Model file for the job. Use its own axes, mm. Give positions to 0.01 mm unless a question says otherwise; leave off trailing zeros. Loops run counter-clockwise (first coordinate to the right, second up) from the corner with the lowest first, then second, coordinate; pieces in that order, holes last. Notation, with made-up numbers: (-39, 28.5) - (-11, 28.5) arc R19 ccw to (-11, 48.5) - close; hole circle Ø4 at (-8, 0.25). An arc over 180 degrees is marked (long way). Use a Markdown table: item, result.
from build123d import *

# Parameters (mm, degrees)
SKETCH_1_R      = 2.5
EXTRUDE_1_DEPTH = 110
SKETCH_2_R      = 2.5
EXTRUDE_2_DEPTH = 7.5


with BuildPart() as part:
    # 草图1 → 凸台-拉伸1 (new, symmetric)
    with BuildSketch(Plane.XY):
        Circle(SKETCH_1_R)
    extrude(amount=EXTRUDE_1_DEPTH, both=True)

    # 草图2 → 凸台-拉伸2 (add)
    with BuildSketch(Plane(origin=(0, 0, 0), x_dir=(0, 0, -1), z_dir=(1, 0, 0))):
        with Locations(Location((-112.44047791, 0, 0), (0, 0, 12.527723759))):
            Circle(SKETCH_2_R)
    extrude_2 = extrude(amount=EXTRUDE_2_DEPTH)

    # 镜向1: 凸台-拉伸2 across plane
    add(extrude_2.mirror(Plane(origin=(0, 0, 0), x_dir=(0, 0, 1), z_dir=(1, 0, 0))))


solid = part.part
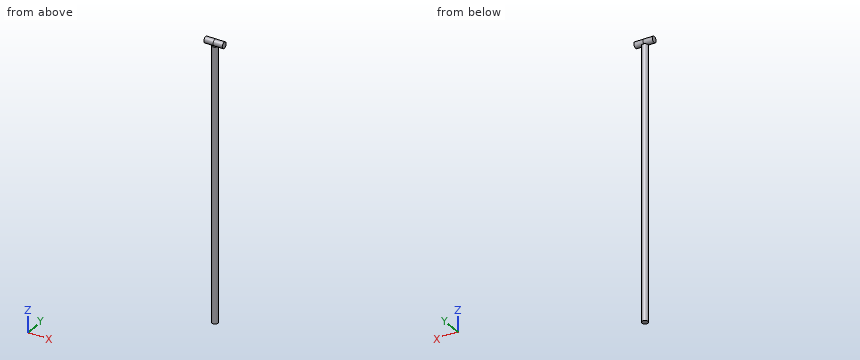
(1) Drill centre lines: probe 1 along X at (y, z) = (-0.2, 45); probe 2 along Z at (x, y) = (0.5, -0.15). Where is each one in solid material? Low to high. Write a range as [from, to].
Computed:
| item | result |
|---|---|
| probe 1 | [-2.49, 2.49] |
| probe 2 | [-110, 114.94] |
(2) Slice it at C-C, the plane x = 4.5. Write the cut outline in (y, z).
Computed:
| item | result |
|---|---|
| outline | circle Ø5 at (0, 112.44) |
(3) Slice it at A-A, the plane y = -1.35. Write the cut outline in (x, z), plus the area to 3 significant figures.
Computed:
| item | result |
|---|---|
| outline | (-7.5, 110.34) - (7.5, 110.34) - (7.5, 114.54) - (-7.5, 114.54) - close; (-2.1, -110) - (2.1, -110) - (2.1, 110) - (-2.1, 110) - close |
| area | 989 mm² |
(4) Slice it at B-B, the plane z = 30.5. Write the cut outline in (x, y).
Computed:
| item | result |
|---|---|
| outline | circle Ø5 at (0, 0) |
(5) Pin check, flat tips, straight feed: P1, Ø1.6, axis at x = 0.5, y = 1, coming from the +Z side; P2, Ø1, axis at x = 0, y = -1.5, coming from the +Z side; P3, Ø2, axis at x = 2.5, z = -21.5, coming from the -Y side; P4, Ø5, axis at x = -1.5, z = -48.5, coming from the +Y side. Stop position of each tip, or through.
Computed:
| item | result |
|---|---|
| P1 | z = 114.93 |
| P2 | z = 114.73 |
| P3 | y = -2 |
| P4 | y = 2.5 |
